```python
from build123d import *

# Parameters (mm, degrees)
SKETCH2_R           = 15.875
BOSS_EXTRUDE1_DEPTH = 25.4
BOSS_EXTRUDE2_DEPTH = 44.45
BOSS_EXTRUDE3_DEPTH = 12.7


with BuildPart() as part:
    # Sketch2 → Boss-Extrude1 (new body)
    with BuildSketch(Plane(origin=(0, 0, 0), x_dir=(1, 0, 0), z_dir=(0, 1, 0))):
        with BuildLine():
            Line((-133.35, 0), (133.35, 0))
            Line((133.35, 0), (133.35, -76.2))
            ThreePointArc((133.35, -76.2), (101.6, -107.95), (69.85, -76.2))
            ThreePointArc((69.85, -76.2), (60.550640303, -53.749359697), (38.1, -44.45))
            Line((38.1, -44.45), (-38.1, -44.45))
            ThreePointArc((-38.1, -44.45), (-60.550640303, -53.749359697), (-69.85, -76.2))
            ThreePointArc((-69.85, -76.2), (-101.6, -107.95), (-133.35, -76.2))
            Line((-133.35, -76.2), (-133.35, 0))
        make_face()
        with Locations((101.6, -76.2)):
            Circle(SKETCH2_R, mode=Mode.SUBTRACT)
        with Locations((-101.6, -76.2)):
            Circle(SKETCH2_R, mode=Mode.SUBTRACT)
    extrude(amount=BOSS_EXTRUDE1_DEPTH)

    # Sketch3 → Boss-Extrude2 (add)
    with BuildSketch(Plane(origin=(0, 0, 0), x_dir=(-1, 0, 0), z_dir=(0, 0, -1))):
        with BuildLine():
            ThreePointArc((63.5, 127), (0, 63.5), (-63.5, 127))
            Line((-63.5, 127), (-88.9, 127))
            Line((-88.9, 127), (-88.9, 57.15))
            ThreePointArc((-88.9, 57.15), (-98.199359697, 34.699359697), (-120.65, 25.4))
            Line((-120.65, 25.4), (0, 25.4))
            Line((0, 25.4), (120.65, 25.4))
            ThreePointArc((120.65, 25.4), (98.199359697, 34.699359697), (88.9, 57.15))
            Line((88.9, 57.15), (88.9, 127))
            Line((88.9, 127), (63.5, 127))
        make_face()
    extrude(amount=-BOSS_EXTRUDE2_DEPTH)

    # Sketch4 → Boss-Extrude3 (add)
    with BuildSketch(Plane(origin=(0, 0, 0), x_dir=(-1, 0, 0), z_dir=(0, 0, -1))):
        with BuildLine():
            Line((-47.625, 127), (-63.5, 127))
            ThreePointArc((-63.5, 127), (0, 63.5), (63.5, 127))
            Line((63.5, 127), (47.625, 127))
            ThreePointArc((47.625, 127), (0, 79.375), (-47.625, 127))
        make_face()
    extrude(amount=-BOSS_EXTRUDE3_DEPTH)


solid = part.part
```
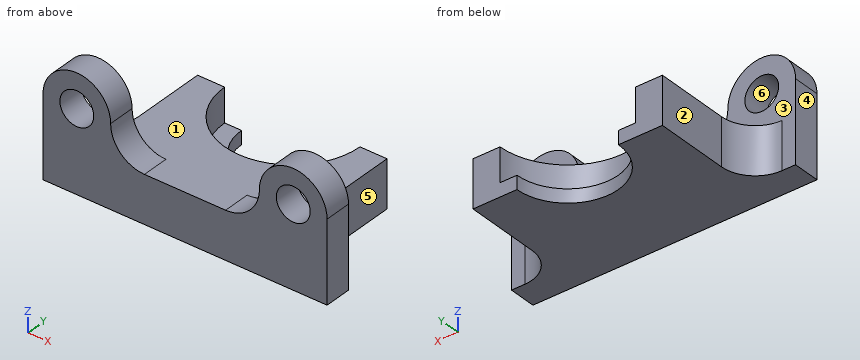
Part model, mm, in its own coordinate system. Face numbers are marked on the shaded views. A direction names the side the tool comes from. Round coordinates to 2 decimals unless told otherwise and drop trailing zeros. Order: outer loops, then holes, each group sorted by start corner. A loop starts at its lowest first (then second) coordinate and runs counter-clockwise, first axis right, second up. Notation, with made-up numbers: M 77,83 L 81,83 A21 cw 81,107 Z; hole C 61.5,0 d6. An arc over 180 degrees is marked long. Answer in a Markdown table with one row per item. Add a question column.
Q1. Cut at A-A on x = 101.6. Give the cut face in (y, z) (3 decimals), and give its area (3 significant figures).
Q2. Cut at C-C on z = 21.5. Give the cut face in (x, y).
Q3. Cut at D-D on z = 99.5. Give the cut face in (x, y), and give its area (3 significant figures).
Q4. Mould opens along X. For the marked faces 4, 5 and 6 say: +X half, -X half, draft (parallel to the pull), parting line (faces both ways), or undercut.
Q5. Cut at B-B on y = 9. Give the cut face in (x, z) (3 decimals).
Q6. Pin check, flat tips, straight feed: pin 1 (2 mm diameter, centred on x = -47.5, y = 55.5, fed in from -Z); pin 2 (22 mm diameter, centred on y = 92, z = 16.5, fed in from +X); pin 3 (4 mm diameter, centred on y = 52, z = 14, fed in from -X); pin 4 (5 mm diameter, centred on x = -15.5, y = 13, fed in from +Z). Stop position of each tip, or through.
Q7. 3-axis set-ups, long thin cutter, end or side, ignore diameter. For the marked faces 1, 2 and 3: which of +Z, -Z, +X, -X, +Y, -Y reach the whole face in a straight line?
Q8. Wall check: L1, parallel to X at y = 5, z = 76; L2, parallel to X at y = 15, z = 76.2 (3 decimals); L3, parallel to Z at x = -101.6, y = 19.75 (3 decimals). Give the ranges that are in metal, low to high. Write a range as from..to.
Established:
| question | item | result |
|---|---|---|
| 1 | outline | M 0,0 L 31.75,0 L 31.75,44.45 L 25.4,44.45 L 25.4,60.325 L 0,60.325 Z; M 0,92.075 L 25.4,92.075 L 25.4,107.95 L 0,107.95 Z |
| 1 | area | 2,220 mm2 |
| 2 | outline | M -133.35,0 L 133.35,0 L 133.35,25.4 L 120.65,25.4 A31.75 cw 88.9,57.15 L 88.9,127 L 63.5,127 A63.5 cw -63.5,127 L -88.9,127 L -88.9,57.15 A31.75 cw -120.65,25.4 L -133.35,25.4 Z |
| 3 | outline | M -123.17,0 L -80.03,0 L -80.03,25.4 L -123.17,25.4 Z; M 80.03,0 L 123.17,0 L 123.17,25.4 L 80.03,25.4 Z |
| 3 | area | 2,190 mm2 |
| 4 | face 4 | -X half |
| 4 | face 5 | +X half |
| 4 | face 6 | undercut |
| 5 | outline | M -133.35,0 L 133.35,0 L 133.35,76.2 A31.75 ccw 69.85,76.2 A31.75 cw 38.1,44.45 L -38.1,44.45 A31.75 cw -69.85,76.2 A31.75 ccw -133.35,76.2 Z; hole C -101.6,76.2 d31.75; hole C 101.6,76.2 d31.75 |
| 6 | pin 1 | stops at z = 0 |
| 6 | pin 2 | stops at x = 88.9 |
| 6 | pin 3 | stops at x = -89.72 |
| 6 | pin 4 | stops at z = 44.45 |
| 7 | face 1 | +Z, +Y |
| 7 | face 2 | +Z, -Z, -X, +Y |
| 7 | face 3 | +Z, -X, +Y |
| 8 | L1 | x = -133.35..-117.47, -85.73..-69.85, 69.85..85.73, 117.47..133.35 |
| 8 | L2 | x = -133.35..-117.475, -85.725..-69.85, 69.85..85.725, 117.475..133.35 |
| 8 | L3 | z = 0..60.325, 92.075..107.95 |
